Read the model definition and answer for the solid it produces. Units are mm, in the model's axes. A direction names the side the tool comes from. Round coordinates to 2 decimals unless told otherwise and drop trailing zeros. Write each loop counter-clockwise with the first axis right and the second up, starting at its lowest first coordinate (ties: lowest second). Pieces come first, ordered by that corner, then holes. Notation, with made-up numbers: M 15.5,-14.5 L 36.5,-14.5 A22 ccw 36.5,12.5 Z; hole C 38.25,-18.5 d3. An arc over 180 degrees is marked long. Use one line per item in the form item = value. Start each with the question number.
```python
from build123d import *

# Parameters (mm, degrees)
F0_W     = 60
F0_H     = 20
F1_DEPTH = 120
F2_W     = 60
F2_H     = 3.121510148
F3_DEPTH = 1
F4_W     = 2
F4_H     = 21.938483119
F5_DEPTH = 1
F6_W     = 10
F6_H     = 6
F7_DEPTH = 5
F8_W     = 10
F8_H     = 6
F9_DEPTH = 5


with BuildPart() as f1:
    # F0 (on Front) → F1 (new body)
    with BuildSketch(Plane.XZ):
        with Locations((30, 10)):
            Rectangle(F0_W, F0_H)
    extrude(amount=F1_DEPTH)

    # F2 (on face) → F3 (cut)
    with BuildSketch(Plane.XY.offset(20)):
        with Locations((30, -96.500761807)):
            Rectangle(F2_W, F2_H)
    extrude(amount=-F3_DEPTH, mode=Mode.SUBTRACT)

    # F4 (on face) → F5 (cut)
    with BuildSketch(Plane.XY.offset(20)):
        with Locations((36.0219793618, -109.0307584405)):
            Rectangle(F4_W, F4_H)
        with Locations((22.2871395051, -109.0307584405)):
            Rectangle(F4_W, F4_H)
    extrude(amount=-F5_DEPTH, mode=Mode.SUBTRACT)

    # F6 (on face) → F7 (cut)
    with BuildSketch(Plane.YZ.offset(60)):
        with Locations((-60, 10)):
            Rectangle(F6_W, F6_H)
    extrude(amount=-F7_DEPTH, mode=Mode.SUBTRACT)

    # F8 (on face) → F9 (cut)
    with BuildSketch(Plane(origin=(0, 0, 0), x_dir=(0, -1, 0), z_dir=(-1, 0, 0))):
        with Locations((60, 10)):
            Rectangle(F8_W, F8_H)
    extrude(amount=-F9_DEPTH, mode=Mode.SUBTRACT)


solid = f1.part
```
Q1. Find section A-A on y = -61. Write down the section's boundary in (x, z).
Q2. A tool of negligible diameter and unlimited length cuts with its end or side. For faces 4 (the face through (2, -60, 13)), 5 (the face through (30, 0, 10)), 6 (the face through (58, -65, 10)), from which of +Z, -Z, +X, -X, +Y, -Y can it reach the whole face along a straight path? Write none if from no direction.
Q3. For a pull along X with two mould halves and no side action, classify faces 1 (the face through (60, -59, 14)), 2 (the face through (2, -65, 10)), 3 (the face through (30, -97, 19)) as +X half, -X half, draft (parallel to the pull), parting line (faces both ways), or undercut.
Q4. Each of these flat-tipped pins is pushed along its axis until it touches: pin 1 Ø1.1 at (x, z) = (11.5, 19.5) entering from +Y; pin 2 Ø5 at (y, z) = (-60.5, 10) entering from -X. Where does it stop, or does it pass through?
Response:
q1.outline = M 0,0 L 60,0 L 60,7 L 55,7 L 55,13 L 60,13 L 60,20 L 0,20 L 0,13 L 5,13 L 5,7 L 0,7 Z
q2.face_4 = -X
q2.face_5 = +Z, -Z, +X, -X, +Y
q2.face_6 = +X
q3.face_1 = +X half
q3.face_2 = draft
q3.face_3 = undercut
q4.pin_1 = 0
q4.pin_2 = 5
